Design review of the part built by this model. Coordinates are the model's own, in mm. A direction names the side the tool comes from. Give positions to 0.01 mm unless a question says otherwise; leave off trailing zeros. Order: outer loops, then holes, each group sorted by start corner. A loop starts at its lowest first (then second) coordinate and runs counter-clockwise, first axis right, second up.
```python
from build123d import *

# Parameters (mm, degrees)
SKETCH3_W           = 32
SKETCH3_H           = 64
BOSS_EXTRUDE2_DEPTH = 3.2
SKETCH4_R           = 2.45
BOSS_EXTRUDE3_DEPTH = 1.8
SKETCH5_W           = 29
SKETCH5_H           = 61
CUT_EXTRUDE1_DEPTH  = 2
SKETCH6_R           = 3.2
BOSS_EXTRUDE4_DEPTH = 2
SKETCH7_R           = 2.5
SKETCH7_R_2         = 2.513496794
CUT_EXTRUDE2_DEPTH  = 2


with BuildPart() as part:
    # Sketch3 → Boss-Extrude2 (new body)
    with BuildSketch(Plane(origin=(0, 0, 0), x_dir=(1, 0, 0), z_dir=(0, 1, 0))):
        Rectangle(SKETCH3_W, SKETCH3_H)
    extrude(amount=BOSS_EXTRUDE2_DEPTH)

    # Sketch4 → Boss-Extrude3 (add)
    with BuildSketch(Plane(origin=(0, 3.2, 0), x_dir=(1, 0, 0), z_dir=(0, 1, 0))):
        with Locations((-12, 28)):
            Circle(SKETCH4_R)
        with Locations((-4, 27.908524957)):
            Circle(SKETCH4_R)
        with Locations((4, 27.908524957)):
            Circle(SKETCH4_R)
        with Locations((12, 28)):
            Circle(SKETCH4_R)
        with Locations((12, 20)):
            Circle(SKETCH4_R)
        with Locations((4, 20)):
            Circle(SKETCH4_R)
        with Locations((-4, 20)):
            Circle(SKETCH4_R)
        with Locations((-12, 20)):
            Circle(SKETCH4_R)
        with Locations((12, 12)):
            Circle(SKETCH4_R)
        with Locations((12, 3.817049914)):
            Circle(SKETCH4_R)
        with Locations((4, 3.908524957)):
            Circle(SKETCH4_R)
        with Locations((4, 11.908524957)):
            Circle(SKETCH4_R)
        with Locations((-4, 11.908524957)):
            Circle(SKETCH4_R)
        with Locations((-4, 3.908524957)):
            Circle(SKETCH4_R)
        with Locations((-12, 3.817049914)):
            Circle(SKETCH4_R)
        with Locations((-12, 12)):
            Circle(SKETCH4_R)
        with Locations((4, -27.908524957)):
            Circle(SKETCH4_R)
        with Locations((12, -28)):
            Circle(SKETCH4_R)
        with Locations((12, -20)):
            Circle(SKETCH4_R)
        with Locations((4, -20)):
            Circle(SKETCH4_R)
        with Locations((4, -11.908524957)):
            Circle(SKETCH4_R)
        with Locations((12, -12)):
            Circle(SKETCH4_R)
        with Locations((12, -3.817049914)):
            Circle(SKETCH4_R)
        with Locations((4, -3.908524957)):
            Circle(SKETCH4_R)
        with Locations((-4, -3.908524957)):
            Circle(SKETCH4_R)
        with Locations((-4, -11.908524957)):
            Circle(SKETCH4_R)
        with Locations((-4, -20)):
            Circle(SKETCH4_R)
        with Locations((-4, -27.908524957)):
            Circle(SKETCH4_R)
        with Locations((-12, -28)):
            Circle(SKETCH4_R)
        with Locations((-12, -20)):
            Circle(SKETCH4_R)
        with Locations((-12, -12)):
            Circle(SKETCH4_R)
        with Locations((-12, -3.817049914)):
            Circle(SKETCH4_R)
    extrude(amount=BOSS_EXTRUDE3_DEPTH)

    # Sketch5 → Cut-Extrude1 (cut)
    with BuildSketch(Plane.XZ):
        Rectangle(SKETCH5_W, SKETCH5_H)
    extrude(amount=-CUT_EXTRUDE1_DEPTH, mode=Mode.SUBTRACT)

    # Sketch6 → Boss-Extrude4 (add)
    with BuildSketch(Plane.XZ.offset(-2)):
        with Locations((-8, 24)):
            Circle(SKETCH6_R)
        with Locations((0, 24)):
            Circle(SKETCH6_R)
        with Locations((8, 24)):
            Circle(SKETCH6_R)
        with Locations((8, 16)):
            Circle(SKETCH6_R)
        with Locations((0, 16)):
            Circle(SKETCH6_R)
        with Locations((-8, 16)):
            Circle(SKETCH6_R)
        with Locations((0, 8)):
            Circle(SKETCH6_R)
        with Locations((8, 8)):
            Circle(SKETCH6_R)
        with Locations((8, 0)):
            Circle(SKETCH6_R)
        Circle(SKETCH6_R)
        with Locations((-8, 0)):
            Circle(SKETCH6_R)
        with Locations((-8, 8)):
            Circle(SKETCH6_R)
        with Locations((8, -24)):
            Circle(SKETCH6_R)
        with Locations((8, -16)):
            Circle(SKETCH6_R)
        with Locations((8, -8)):
            Circle(SKETCH6_R)
        with Locations((0, -8)):
            Circle(SKETCH6_R)
        with Locations((0, -16)):
            Circle(SKETCH6_R)
        with Locations((0, -24)):
            Circle(SKETCH6_R)
        with Locations((-8, -24)):
            Circle(SKETCH6_R)
        with Locations((-8, -16)):
            Circle(SKETCH6_R)
        with Locations((-8, -8)):
            Circle(SKETCH6_R)
    extrude(amount=BOSS_EXTRUDE4_DEPTH)

    # Sketch7 → Cut-Extrude2 (cut)
    with BuildSketch(Plane.XZ.offset(-2)):
        with Locations((-8, -24)):
            Circle(SKETCH7_R)
        with Locations((0, -24)):
            Circle(SKETCH7_R)
        with Locations((8, -24)):
            Circle(SKETCH7_R_2)
        with Locations((-8, -16)):
            Circle(SKETCH7_R)
        with Locations((0, -16)):
            Circle(SKETCH7_R)
        with Locations((8, -16)):
            Circle(SKETCH7_R)
        with Locations((-8, -8)):
            Circle(SKETCH7_R)
        with Locations((0, -8)):
            Circle(SKETCH7_R)
        with Locations((8, -8)):
            Circle(SKETCH7_R)
        with Locations((-8, 8)):
            Circle(SKETCH7_R)
        with Locations((0, 8)):
            Circle(SKETCH7_R)
        with Locations((8, 8)):
            Circle(SKETCH7_R_2)
        with Locations((8, 0)):
            Circle(SKETCH7_R)
        Circle(SKETCH7_R)
        with Locations((-8, 0)):
            Circle(SKETCH7_R)
        with Locations((0, 16)):
            Circle(SKETCH7_R)
        with Locations((8, 16)):
            Circle(SKETCH7_R)
        with Locations((8, 24)):
            Circle(SKETCH7_R)
        with Locations((0, 24)):
            Circle(SKETCH7_R)
        with Locations((-8, 24)):
            Circle(SKETCH7_R)
        with Locations((-8, 16)):
            Circle(SKETCH7_R)
    extrude(amount=CUT_EXTRUDE2_DEPTH, mode=Mode.SUBTRACT)


solid = part.part
```
1. Take a section at A-A (z = -20). State the section outline as (x, y) points, then the cut area to 3 significant figures.
Recorded:
outline: (-16, 0) - (-14.5, 0) - (-14.5, 2) - (14.5, 2) - (14.5, 0) - (16, 0) - (16, 3.2) - (14.45, 3.2) - (14.45, 5) - (9.55, 5) - (9.55, 3.2) - (6.45, 3.2) - (6.45, 5) - (1.55, 5) - (1.55, 3.2) - (-1.55, 3.2) - (-1.55, 5) - (-6.45, 5) - (-6.45, 3.2) - (-9.55, 3.2) - (-9.55, 5) - (-14.45, 5) - (-14.45, 3.2) - (-16, 3.2) - close
area: 79.7 mm2
2. Take a section at B-B (y = 4.25). State how many separate pieces and enclosed holes the cut face has, then the cut area to 3 significant figures.
Recorded:
separate pieces: 32
enclosed holes: 0
area: 603 mm2
3. For line 1 along X through (y, z) = (1, -28); line 2 along Y through (x, z) = (-4, 28); line 3 along Y through (x, z) = (6.5, -27), list the stretches that pass through material, from the lowest coordinate up.
Recorded:
line 1: x = -16 to -14.5, 14.5 to 16
line 2: y = 2 to 5
line 3: y = 2 to 3.2
4. For pin 1 (2.5 mm diameter, centred on x = 8, z = -24.5, fed in from -Y); pin 2 (8 mm diameter, centred on x = 8, z = 24, fed in from +Y); pin 3 (4 mm diameter, centred on x = -8, z = -16, fed in from +Y), all flat-tipped, find the tip position at first contact; note any pin that passes through.
Recorded:
pin 1: stops at y = 2
pin 2: stops at y = 5
pin 3: stops at y = 3.2
5. Draft analysis for pull direction Z (two halves, no side actions). For faces 4 (the face through (-12.32, 4.09, 25.57)), 5 (the face through (-2, 0, 22)), 6 (the face through (0, 2, 16)), state which applies: pulls with the +Z half, pulls with the -Z half, needs draft (parallel to the pull), parting line crosses it, or undercut.
Recorded:
face 4: undercut
face 5: needs draft
face 6: undercut
6. Machinability: for faces 1 (the face through (-4.53, 4.09, 14.3)), 2 (the face through (10.322, 1.014, 7.037)), 3 (the face through (-4, 5, 20)), which of the approach directions +Z, -Z, +X, -X, +Y, -Y give a long, thin tool a straight path to every point of the face, cutting with its end or side? Answer none if there is none.
Recorded:
face 1: +Y
face 2: -Y
face 3: +Z, -Z, +X, -X, +Y
